from build123d import *

# Parameters (mm, degrees)
F1_DEPTH = 5
F2_DEPTH = 10
F0_W     = 80
F0_H     = 80
F3_DEPTH = 20
F4_DEPTH = 5


with BuildPart() as f1:
    # F0 (on Front) → F1 (new body)
    with BuildSketch(Plane.XZ):
        with BuildLine():
            Line((-21, 65), (-49, 65))
            ThreePointArc((-49, 65), (-53.242641, 63.242641), (-55, 59))
            Line((-55, 59), (-55, 31))
            ThreePointArc((-55, 31), (-53.242641, 26.757359), (-49, 25))
            Line((-49, 25), (-21, 25))
            ThreePointArc((-21, 25), (-16.757359, 26.757359), (-15, 31))
            Line((-15, 31), (-15, 59))
            ThreePointArc((-15, 59), (-16.757359, 63.242641), (-21, 65))
        make_face()
    extrude(amount=F1_DEPTH)

    # F0 (on Front) → F2 (join)
    with BuildSketch(Plane.XZ):
        with BuildLine():
            Line((-15, 75), (-55, 75))
            ThreePointArc((-55, 75), (-62.071068, 72.071068), (-65, 65))
            Line((-65, 65), (-65, 25))
            ThreePointArc((-65, 25), (-62.071068, 17.928932), (-55, 15))
            Line((-55, 15), (-15, 15))
            ThreePointArc((-15, 15), (-7.928932, 17.928932), (-5, 25))
            Line((-5, 25), (-5, 65))
            ThreePointArc((-5, 65), (-7.928932, 72.071068), (-15, 75))
        make_face()
        with BuildLine():
            ThreePointArc((-55, 59), (-53.242641, 63.242641), (-49, 65))
            Line((-49, 65), (-21, 65))
            ThreePointArc((-21, 65), (-16.757359, 63.242641), (-15, 59))
            Line((-15, 59), (-15, 31))
            ThreePointArc((-15, 31), (-16.757359, 26.757359), (-21, 25))
            Line((-21, 25), (-49, 25))
            ThreePointArc((-49, 25), (-53.242641, 26.757359), (-55, 31))
            Line((-55, 31), (-55, 59))
        make_face(mode=Mode.SUBTRACT)
    extrude(amount=F2_DEPTH)

    # F0 (on Front) → F3 (join)
    with BuildSketch(Plane.XZ):
        with Locations((-40, 40)):
            Rectangle(F0_W, F0_H)
        with BuildLine():
            ThreePointArc((-68, 25), (-74.828427, 22.171573), (-72, 29))
            ThreePointArc((-72, 29), (-69.171573, 27.828427), (-68, 25))
        make_face(mode=Mode.SUBTRACT)
        with BuildLine():
            ThreePointArc((-72, 61), (-74.828427, 67.828427), (-68, 65))
            ThreePointArc((-68, 65), (-69.171573, 62.171573), (-72, 61))
        make_face(mode=Mode.SUBTRACT)
        with BuildLine():
            ThreePointArc((-65, 65), (-62.071068, 72.071068), (-55, 75))
            Line((-55, 75), (-15, 75))
            ThreePointArc((-15, 75), (-7.928932, 72.071068), (-5, 65))
            Line((-5, 65), (-5, 25))
            ThreePointArc((-5, 25), (-7.928932, 17.928932), (-15, 15))
            Line((-15, 15), (-55, 15))
            ThreePointArc((-55, 15), (-62.071068, 17.928932), (-65, 25))
            Line((-65, 25), (-65, 65))
        make_face(mode=Mode.SUBTRACT)
    extrude(amount=F3_DEPTH)

    # F0 (on Front) → F4 (join)
    with BuildSketch(Plane.XZ):
        with BuildLine():
            ThreePointArc((-72, 61), (-69.171573, 62.171573), (-68, 65))
            ThreePointArc((-68, 65), (-74.828427, 67.828427), (-72, 61))
        make_face()
        with BuildLine():
            ThreePointArc((-68, 25), (-69.171573, 27.828427), (-72, 29))
            ThreePointArc((-72, 29), (-74.828427, 22.171573), (-68, 25))
        make_face()
    extrude(amount=F4_DEPTH)


solid = f1.part
Part model, mm, in its own coordinate system. A direction names the side the tool comes from. Coordinates: 2 decimals unless noted, no trailing zeros. Order: outer loops, then holes, each group sorted by start corner. A loop starts at its lowest first (then second) coordinate and runs counter-clockwise, first axis right, second up. Notation, with made-up numbers: M 26,5 L 83,5 A28 cw 83,24 Z; hole C -30,-37.75 d1. An arc over 180 degrees is marked long. One line per question, with ' | ' between items.
Q1. Slice it at C-C (x = -35.5). Give the cut face in (y, z), and give its area (3 significant figures).
A:
outline: M -20,0 L 0,0 L 0,80 L -20,80 L -20,75 L -10,75 L -10,65 L -5,65 L -5,25 L -10,25 L -10,15 L -20,15 Z | area: 800 mm^2
Q2. Pin check, flat tips, straight feed: P1, Ø1, axis at x = -51, z = 61.5, coming from the -Y side; P2, Ø18, axis at x = -49.5, z = 35, coming from the -Y side. Stop position of each tip, or through.
A:
P1: stops at y = -5 | P2: stops at y = -10
Q3. Drill centre lines: line 1 (Z direction, x = -72, y = -13.5); line 2 (X direction, y = -17, z = 25); line 3 (Z direction, x = -53, y = -18.5). Where is each one in solid material? Low to high.
A:
line 1: z = 0 to 21, 29 to 61, 69 to 80 | line 2: x = -80 to -76, -68 to -65, -5 to 0 | line 3: z = 0 to 15, 75 to 80
Q4. Slice it at A-A (y = -14.25). Give the cut face in (x, z), and give its area (3 significant figures).
A:
outline: M -80,0 L 0,0 L 0,80 L -80,80 Z; hole C -72,25 d8; hole C -72,65 d8; hole M -65,25 A10 ccw -55,15 L -15,15 A10 ccw -5,25 L -5,65 A10 ccw -15,75 L -55,75 A10 ccw -65,65 Z | area: 2,790 mm^2
Q5. Slice it at B-B (z = 73). Give the cut face in (x, y), and give its area (3 significant figures).
A:
outline: M -80,-20 L -61,-20 L -61,-10 L -9,-10 L -9,-20 L 0,-20 L 0,0 L -80,0 Z | area: 1,080 mm^2
Q6. Slice it at D-D (y = -7.5). Give the cut face in (x, z).
A:
outline: M -80,0 L 0,0 L 0,80 L -80,80 Z; hole C -72,25 d8; hole C -72,65 d8; hole M -55,31 A6 ccw -49,25 L -21,25 A6 ccw -15,31 L -15,59 A6 ccw -21,65 L -49,65 A6 ccw -55,59 Z
Q7. 3-axis set-ups, long thin cutter, end or side, ignore diameter. For faces 1 (the face through (-53.289, -7.465, 63.196)), 2 (the face through (-67, -20, 41)): which of +Z, -Z, +X, -X, +Y, -Y reach the whole face in a straight line?
A:
face 1: -Y | face 2: +Z, -Z, +X, -X, -Y
